Verification items for the finished model (mm, model axes). Face numbers are marked on the shaded views. Give positions to 0.01 mm unless a question says otherwise; leave off trailing zeros. Write each loop counter-clockwise with the first axis right and the second up, starting at its lowest first coordinate (ties: lowest second). Pieces come first, ordered by that corner, then holes. Notation, with made-up numbers: (89, 64.25) -> (135, 64.25) arc R30 cw to (135, 102.25) -> close; hole circle Ø9 at (-38, 18.25). An arc over 180 degrees is marked (long way). Write item = value, one per line.
from build123d import *

# Parameters (mm, degrees)
F0_R     = 2.75
F0_R_2   = 16
F1_DEPTH = 20
F2_R     = 3.3
F3_DEPTH = 38
F4_R     = 5.5
F5_DEPTH = 4
F6_SIZE  = 2


with BuildPart() as f1:
    # F0 (on Front) → F1 (new body)
    with BuildSketch(Plane.XZ):
        Polygon((0, 70), (0, 0), (38, 0), (38, 15), (48, 15), (48, 55), (38, 55), (38, 70), align=None)
        with Locations((10, 8)):
            Circle(F0_R, mode=Mode.SUBTRACT)
        with Locations((28, 8)):
            Circle(F0_R, mode=Mode.SUBTRACT)
        with Locations((10, 62)):
            Circle(F0_R, mode=Mode.SUBTRACT)
        with Locations((28, 35)):
            Circle(F0_R_2, mode=Mode.SUBTRACT)
        with Locations((28, 62)):
            Circle(F0_R, mode=Mode.SUBTRACT)
    extrude(amount=F1_DEPTH)

    # F2 (on face) → F3 (cut)
    with BuildSketch(Plane.YZ.offset(38)):
        with Locations((-10, 62)):
            Circle(F2_R)
        with Locations((-10, 8)):
            Circle(F2_R)
    extrude(amount=-F3_DEPTH, mode=Mode.SUBTRACT)

    # F4 (on face) → F5 (cut)
    with BuildSketch(Plane.YZ.offset(38)):
        with Locations((-10, 62)):
            Circle(F4_R)
        with Locations((-10, 8)):
            Circle(F4_R)
    extrude(amount=-F5_DEPTH, mode=Mode.SUBTRACT)

    # F6
    f6_edges = [f1.edges().sort_by_distance(p)[0] for p in [
        (38, -10, 70),
        (48, -10, 55),
        (38, -10, 0),
        (48, -10, 15),
    ]]
    chamfer(f6_edges, length=F6_SIZE)


solid = f1.part
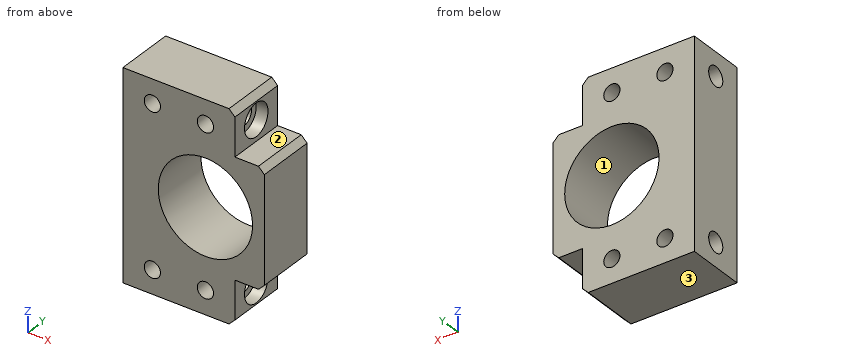
Item 1: Sectioned sample at D-D on x = 10. Record the cut outline in (y, z), then the cut area to 3 significant figures.
Response values:
outline = (-20, 0) -> (0, 0) -> (0, 5.25) -> (-8.18, 5.25) arc R3.3 cw to (-11.82, 5.25) -> (-20, 5.25) -> close; (-20, 10.75) -> (-11.82, 10.75) arc R3.3 cw to (-8.18, 10.75) -> (0, 10.75) -> (0, 59.25) -> (-8.18, 59.25) arc R3.3 cw to (-11.82, 59.25) -> (-20, 59.25) -> close; (-20, 64.75) -> (-11.82, 64.75) arc R3.3 cw to (-8.18, 64.75) -> (0, 64.75) -> (0, 70) -> (-20, 70) -> close
area = 1,170 mm^2
Item 2: Mould release check, pull along Z, two halves, no side actions. Record for the marked faces 1, 2 and 3: +Z half, -Z half, draft (parallel to the pull), parting line (faces both ways), or undercut.
Response values:
face_1 = undercut
face_2 = +Z half
face_3 = -Z half
Item 3: Sectioned sample at C-C on x = 28. Record the cut outline in (y, z).
Response values:
outline = (-20, 0) -> (0, 0) -> (0, 5.25) -> (-8.18, 5.25) arc R3.3 cw to (-11.82, 5.25) -> (-20, 5.25) -> close; (-20, 10.75) -> (-11.82, 10.75) arc R3.3 cw to (-8.18, 10.75) -> (0, 10.75) -> (0, 19) -> (-20, 19) -> close; (-20, 51) -> (0, 51) -> (0, 59.25) -> (-8.18, 59.25) arc R3.3 cw to (-11.82, 59.25) -> (-20, 59.25) -> close; (-20, 64.75) -> (-11.82, 64.75) arc R3.3 cw to (-8.18, 64.75) -> (0, 64.75) -> (0, 70) -> (-20, 70) -> close
Item 4: Sectioned sample at B-B on z = 35. Record the cut outline in (x, y), then the cut area to 3 significant figures.
Response values:
outline = (0, -20) -> (12, -20) -> (12, 0) -> (0, 0) -> close; (44, -20) -> (48, -20) -> (48, 0) -> (44, 0) -> close
area = 320 mm^2
Item 5: Sectioned sample at A-A on y = -10. Give the number of separate pieces and of enclosed holes in the cut face, then the cut area to 3 significant figures.
Response values:
separate_pieces = 3
enclosed_holes = 1
area = 1,710 mm^2
Item 6: Go/stop test with flat-tipped pins: P1, Ø5, axis at y = -13.5, z = 48, coming from the -X side; P2, Ø6.5, axis at y = -8, z = 10, coming from the +X side; P3, Ø5.5, axis at y = -11, z = 62, coming from the +X side. Record where each tip stops, or that it passes through.
Response values:
P1 = 0
P2 = 38
P3 = 34
Item 7: Material ranges on line 1 (Z direction, x = 10, y = -16); line 2 (Z direction, x = 28, y = -14.25); line 3 (X direction, y = -3.5, z = 62), recorded low to high.
Response values:
line_1 = 0 to 5.25, 10.75 to 59.25, 64.75 to 70
line_2 = 0 to 5.25, 10.75 to 19, 51 to 59.25, 64.75 to 70
line_3 = 0 to 7.25, 12.75 to 25.25, 30.75 to 38
